```python
from build123d import *

# Parameters (mm, degrees)
SKETCH1_R           = 12.7
SKETCH1_R_2         = 6.35
BOSS_EXTRUDE1_DEPTH = 3.175
BOSS_EXTRUDE2_DEPTH = 3.175
CIRPATTERN1_COUNT   = 13


with BuildPart() as part:
    # Sketch1 → Boss-Extrude1 (new body)
    with BuildSketch(Plane.XY):
        Circle(SKETCH1_R)
        Circle(SKETCH1_R_2, mode=Mode.SUBTRACT)
    extrude(amount=BOSS_EXTRUDE1_DEPTH)

    # Sketch2 → Boss-Extrude2 (add)
    with BuildSketch(Plane.XY):
        Polygon((-1.27, 15.24), (1.27, 15.24), (1.905, 12.065), (-1.905, 12.065), align=None)
    boss_extrude2 = extrude(amount=BOSS_EXTRUDE2_DEPTH)

    # CirPattern1: Boss-Extrude2 ×13 about axis
    cirpattern1_axis = Axis((0, 0, 0), (0, 0, 1))
    for i in range(1, CIRPATTERN1_COUNT):
        add(boss_extrude2.rotate(cirpattern1_axis, i * 360 / CIRPATTERN1_COUNT))


solid = part.part
```
The model under review builds one solid part; all positions refer to its coordinate system, in mm. A direction names the side the tool comes from. Round coordinates to 2 decimals unless told otherwise and drop trailing zeros. Loops run counter-clockwise (first coordinate to the right, second up) from the corner with the lowest first, then second, coordinate; pieces in that order, holes last. Notation, with made-up numbers: M -19,17 L 32,17 A27 cw 32,48 Z; hole C -24,1.25 d2. An arc over 180 degrees is marked long. Write item = value, one per line.
Item 1: Machinability: for faces 1 (the flat face through (-10.381, -9.406, 1.565)), 2 (the flat face through (1.844, -13.887, 1.565)), 3 (the flat face through (13.6, 3.203, 1.565)), which of the approach directions +Z, -Z, +X, -X, +Y, -Y give a long, thin tool a straight path to every point of the face, cutting with its end or side? Answer none if there is none.
Return value:
face_1 = +Z, -Z, -X
face_2 = +Z, -Z, -Y
face_3 = +Z, -Z, +X
Item 2: Take a section at C-C on y = 11. Write out the cut boundary in (x, z) (3 decimals).
Return value:
outline = M -7.647,0 L 7.647,0 L 7.647,3.175 L -7.647,3.175 Z
Item 3: Take a section at D-D on y = -10. Write out the cut boundary in (x, z) (3 decimals), then the cut area to 3 significant figures.
Return value:
outline = M -10.727,0 L 10.727,0 L 10.727,3.175 L -10.727,3.175 Z
area = 68.1 mm2
Item 4: Take a section at A-A on x = 0. Write out the cut boundary in (y, z) (3 decimals), then the cut area to 3 significant figures.
Return value:
outline = M -12.7,0 L -6.35,0 L -6.35,3.175 L -12.7,3.175 Z; M 6.35,0 L 15.24,0 L 15.24,3.175 L 6.35,3.175 Z
area = 48.4 mm2
Item 5: Insertion check: P1, Ø11.5, axis at x = 0, y = 0, coming from the -Z side. The pin has a flat end and moves straight along its axis. Give the tip position at first contact, or say it passes through.
Return value:
P1 = through
Item 6: For line 1 (Y direction, x = 0, z = 2.5); line 2 (X direction, y = 9, z = 1.4); line 3 (X direction, y = 14, z = 1.85), list the stretches that pass through material, from the lowest coordinate up. Write a range as [from, to].
Return value:
line_1 = [-12.7, -6.35], [6.35, 15.24]
line_2 = [-12.31, -10.19], [-8.96, 8.96], [10.19, 12.31]
line_3 = [-6.12, -5.89], [-1.52, 1.52], [5.89, 6.12]
Item 7: Take a section at B-B on y = -1.5. Write out the cut boundary in (x, z) (3 decimals), then the cut area to 3 significant figures.
Return value:
outline = M -12.611,0 L -6.17,0 L -6.17,3.175 L -12.611,3.175 Z; M 6.17,0 L 12.611,0 L 12.611,3.175 L 6.17,3.175 Z
area = 40.9 mm2
Item 8: The part is to be moulded in two halves that separate along Y. For faces 4 (the cylindrical face through (12.605, -1.548, 1.565)), 5 (the cylindrical face through (0, -12.7, 1.6)), 6 (the flat face through (-3, -6, 0)), say which applies: released by +Y, released by -Y, zero draft, split by the parting line, or undercut.
Return value:
face_4 = undercut
face_5 = released by -Y
face_6 = zero draft
